Read the model definition and answer for the solid it produces. Units are mm, in the model's axes. Round coordinates to 2 decimals unless told otherwise and drop trailing zeros. Loops run counter-clockwise (first coordinate to the right, second up) from the corner with the lowest first, then second, coordinate; pieces in that order, holes last. Notation, with made-up numbers: (6, 6) - (31, 6) arc R26 cw to (31, 43) - close; hole circle Ø9 at (-23.5, 18.5). An arc over 180 degrees is marked (long way). Answer as CSV lines item,"result".
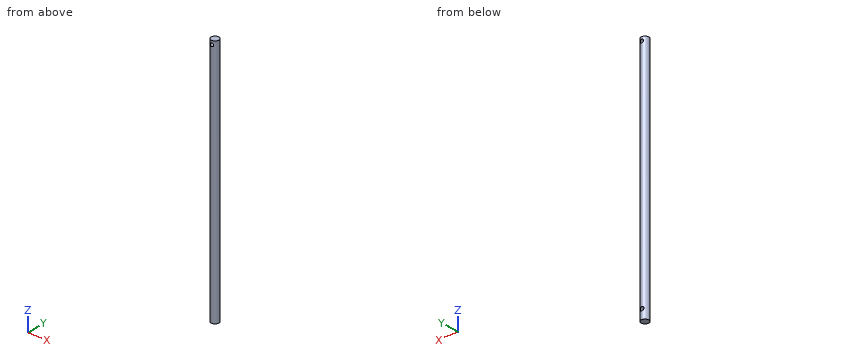
```python
from build123d import *

# Parameters (mm, degrees)
SKETCH_1_R                   = 4
EXTRUDE_1_DEPTH              = 259
HOLE_WIZARD_M4_2_D           = 3.3
HOLE_WIZARD_M4_2_DEPTH       = 6.1
HOLE_WIZARD_M4_2_CBORE_D     = 4
HOLE_WIZARD_M4_2_CBORE_DEPTH = 4
HOLE_WIZARD_M4_2_TIP         = 0.991420021
SKETCH_7_R                   = 1.69
CUT_EXTRUDE_1_DEPTH          = 260.154394241


with BuildPart() as part:
    # 草图1 → 拉伸1 (new body)
    with BuildSketch(Plane.XY):
        Circle(SKETCH_1_R)
    extrude(amount=EXTRUDE_1_DEPTH)

    # M4 螺纹孔2
    with Locations(Plane(origin=(0, 4, 0), x_dir=(-1, 0, 0), z_dir=(0, 1, 0))):
        with Locations((0, 10)):
            CounterBoreHole(HOLE_WIZARD_M4_2_D / 2, HOLE_WIZARD_M4_2_CBORE_D / 2, HOLE_WIZARD_M4_2_CBORE_DEPTH, depth=HOLE_WIZARD_M4_2_DEPTH)
            with Locations((0, 0, -(HOLE_WIZARD_M4_2_DEPTH + HOLE_WIZARD_M4_2_TIP / 2))):  # 118° drill point
                Cone(0, HOLE_WIZARD_M4_2_D / 2, HOLE_WIZARD_M4_2_TIP, mode=Mode.SUBTRACT)

    # 草图7 → 切除-拉伸1 (cut, through all)
    with BuildSketch(Plane(origin=(0, 4, 0), x_dir=(-1, 0, 0), z_dir=(0, 1, 0))):
        with Locations(Location((0, 255, 0), (0, 0, 90))):
            Circle(SKETCH_7_R)
    extrude(amount=-CUT_EXTRUDE_1_DEPTH, mode=Mode.SUBTRACT)


solid = part.part
```
1) Each of these flat-tipped pins is pushed along its axis until it touches: P1, Ø1, axis at y = -1.5, z = 213, coming from the +X side; P2, Ø2, axis at x = -0.5, z = 9.5, coming from the +Y side; P3, Ø4, axis at x = 0.5, z = 119, coming from the +Y side. Where does it stop, or does it pass through?
Entries:
P1,"stops at x = 3.87"
P2,"stops at y = 0"
P3,"stops at y = 4"
2) Find the intervals of material crossed by line 1 (Z direction, x = 0, y = -1); line 2 (Z direction, x = 0, y = 0.5); line 3 (Y direction, x = -0.5, z = 171.5), in increasing order.
Entries:
line 1,"z = 0 to 8.35, 11.65 to 253.31, 256.69 to 259"
line 2,"z = 0 to 8, 12 to 253.31, 256.69 to 259"
line 3,"y = -3.97 to 3.97"
3) A cutting plane is placed at A-A, the plane z = 241.5. Determine the outline of the cut face in (x, y).
Entries:
outline,"circle Ø8 at (0, 0)"
